```python
from build123d import *

# Parameters (mm, degrees)
SKETCH1_R           = 11
SKETCH1_R_2         = 1.5
SKETCH1_R_3         = 4
BOSS_EXTRUDE1_DEPTH = 16
SKETCH1_4_R         = 11
SKETCH1_4_R_2       = 8
BOSS_EXTRUDE2_DEPTH = 9
SKETCH2_R           = 4
CUT_EXTRUDE1_DEPTH  = 204.169017313
SKETCH3_R           = 4
CUT_EXTRUDE2_DEPTH  = 204.169017313
SKETCH1_5_R         = 11
SKETCH1_5_R_2       = 8
BOSS_EXTRUDE3_DEPTH = 9
CUT_EXTRUDE3_DEPTH  = 2.5
SKETCH5_R           = 4
BOSS_EXTRUDE4_DEPTH = 40
SKETCH6_R           = 4
BOSS_EXTRUDE5_DEPTH = 40


with BuildPart() as part:
    # Sketch1 → Boss-Extrude1 (new body)
    with BuildSketch(Plane(origin=(0, 0, 0), x_dir=(1, 0, 0), z_dir=(0, 1, 0))):
        with BuildLine():
            Line((196.404615305, 34.409093194), (187.656854249, 43.156854249))
            ThreePointArc((187.656854249, 43.156854249), (178.938532541, 44.89103626), (174, 37.5))
            Line((174, 37.5), (174, 24))
            ThreePointArc((174, 24), (171.656854249, 18.343145751), (166, 16))
            Line((166, 16), (150, 16))
            ThreePointArc((150, 16), (145.757359313, 14.242640687), (144, 10))
            Line((144, 10), (144, -10))
            ThreePointArc((144, -10), (145.757359313, -14.242640687), (150, -16))
            Line((150, -16), (166, -16))
            ThreePointArc((166, -16), (171.656854249, -18.343145751), (174, -24))
            Line((174, -24), (174, -37.5))
            ThreePointArc((174, -37.5), (178.938532541, -44.89103626), (187.656854249, -43.156854249))
            Line((187.656854249, -43.156854249), (196.404615305, -34.409093194))
            Line((196.404615305, -34.409093194), (209.37167645, -47.376154339))
            Line((209.37167645, -47.376154339), (237.655947698, -19.091883092))
            Line((237.655947698, -19.091883092), (220, -1.435935394))
            Line((220, -1.435935394), (220, 1.435935394))
            Line((220, 1.435935394), (237.655947698, 19.091883092))
            Line((237.655947698, 19.091883092), (209.37167645, 47.376154339))
            Line((209.37167645, 47.376154339), (196.404615305, 34.409093194))
        make_face()
        with Locations(Location((160, 0, 0), (0, 0, 270))):
            Circle(SKETCH1_R, mode=Mode.SUBTRACT)
        with Locations(Location((150, 10, 0), (0, 0, 270))):
            Circle(SKETCH1_R_2, mode=Mode.SUBTRACT)
        with Locations(Location((170, 10, 0), (0, 0, 270))):
            Circle(SKETCH1_R_2, mode=Mode.SUBTRACT)
        with Locations(Location((170, -10, 0), (0, 0, 270))):
            Circle(SKETCH1_R_2, mode=Mode.SUBTRACT)
        with Locations(Location((150, -10, 0), (0, 0, 270))):
            Circle(SKETCH1_R_2, mode=Mode.SUBTRACT)
        with Locations(Location((204, 0, 0), (0, 0, 270))):
            Circle(SKETCH1_R, mode=Mode.SUBTRACT)
        with Locations(Location((182, 37.5, 0), (0, 0, 270))):
            Circle(SKETCH1_R_3, mode=Mode.SUBTRACT)
        with Locations(Location((194, 10, 0), (0, 0, 270))):
            Circle(SKETCH1_R_2, mode=Mode.SUBTRACT)
        with Locations(Location((214, 10, 0), (0, 0, 270))):
            Circle(SKETCH1_R_2, mode=Mode.SUBTRACT)
        with Locations(Location((214, -10, 0), (0, 0, 270))):
            Circle(SKETCH1_R_2, mode=Mode.SUBTRACT)
        with Locations(Location((194, -10, 0), (0, 0, 270))):
            Circle(SKETCH1_R_2, mode=Mode.SUBTRACT)
        with Locations(Location((182, -37.5, 0), (0, 0, 270))):
            Circle(SKETCH1_R_3, mode=Mode.SUBTRACT)
    extrude(amount=BOSS_EXTRUDE1_DEPTH)

    # Sketch1<4> → Boss-Extrude2 (add)
    with BuildSketch(Plane(origin=(0, 0, 0), x_dir=(1, 0, 0), z_dir=(0, 1, 0))):
        with Locations(Location((204, 0, 0), (0, 0, 270))):
            Circle(SKETCH1_4_R)
        with Locations(Location((204, 0, 0), (0, 0, 270))):
            Circle(SKETCH1_4_R_2, mode=Mode.SUBTRACT)
    extrude(amount=BOSS_EXTRUDE2_DEPTH)

    # Sketch2 → Cut-Extrude1 (cut, through all)
    with BuildSketch(Plane(origin=(109.282032303, 0, 109.282032303), x_dir=(0.7071067811865286, 0, -0.7071067811865666), z_dir=(0.7071067811865666, 0, 0.7071067811865286))):
        with Locations((173.548132206, 8)):
            Circle(SKETCH2_R)
    extrude(amount=-CUT_EXTRUDE1_DEPTH, mode=Mode.SUBTRACT)

    # Sketch3 → Cut-Extrude2 (cut, through all)
    with BuildSketch(Plane(origin=(109.282032303, 0, -109.282032303), x_dir=(-0.7071067811865511, 0, -0.707106781186544), z_dir=(0.707106781186544, 0, -0.7071067811865511))):
        with Locations((-173.548132206, 8)):
            Circle(SKETCH3_R)
    extrude(amount=-CUT_EXTRUDE2_DEPTH, mode=Mode.SUBTRACT)

    # Sketch1<5> → Boss-Extrude3 (add)
    with BuildSketch(Plane(origin=(0, 0, 0), x_dir=(1, 0, 0), z_dir=(0, 1, 0))):
        with Locations(Location((160, 0, 0), (0, 0, 270))):
            Circle(SKETCH1_5_R)
        with Locations(Location((160, 0, 0), (0, 0, 270))):
            Circle(SKETCH1_5_R_2, mode=Mode.SUBTRACT)
    extrude(amount=BOSS_EXTRUDE3_DEPTH)

    # Sketch4 → Cut-Extrude3 (cut)
    with BuildSketch(Plane.XZ):
        Polygon((153.464101615, 10), (151.732050808, 13), (148.267949192, 13), (146.535898385, 10), (148.267949192, 7), (151.732050808, 7), align=None)
        Polygon((173.464101615, 10), (171.732050808, 13), (168.267949192, 13), (166.535898385, 10), (168.267949192, 7), (171.732050808, 7), align=None)
        Polygon((153.464101615, -10), (151.732050808, -7), (148.267949192, -7), (146.535898385, -10), (148.267949192, -13), (151.732050808, -13), align=None)
        Polygon((173.464101615, -10), (171.732050808, -7), (168.267949192, -7), (166.535898385, -10), (168.267949192, -13), (171.732050808, -13), align=None)
        Polygon((197.464101615, 10), (195.732050808, 13), (192.267949192, 13), (190.535898385, 10), (192.267949192, 7), (195.732050808, 7), align=None)
        Polygon((217.464101615, 10), (215.732050808, 13), (212.267949192, 13), (210.535898385, 10), (212.267949192, 7), (215.732050808, 7), align=None)
        Polygon((197.464101615, -10), (195.732050808, -7), (192.267949192, -7), (190.535898385, -10), (192.267949192, -13), (195.732050808, -13), align=None)
        Polygon((217.464101615, -10), (215.732050808, -7), (212.267949192, -7), (210.535898385, -10), (212.267949192, -13), (215.732050808, -13), align=None)
    extrude(amount=-CUT_EXTRUDE3_DEPTH, mode=Mode.SUBTRACT)

    # Sketch5 → Boss-Extrude4 (add)
    with BuildSketch(Plane(origin=(80.997761055, 0, -80.997761055), x_dir=(0.7071067811865509, 0, 0.7071067811865441), z_dir=(-0.7071067811865441, 0, 0.7071067811865509))):
        with BuildLine():
            Line((181.548132206, 16), (181.548132206, 23))
            ThreePointArc((181.548132206, 23), (173.548132206, 31), (165.548132206, 23))
            Line((165.548132206, 23), (165.548132206, 16))
            Line((165.548132206, 16), (181.548132206, 16))
        make_face()
        with Locations((173.548132206, 23)):
            Circle(SKETCH5_R, mode=Mode.SUBTRACT)
    extrude(amount=-BOSS_EXTRUDE4_DEPTH)

    # Sketch6 → Boss-Extrude5 (add)
    with BuildSketch(Plane(origin=(80.997761055, 0, 80.997761055), x_dir=(-0.7071067811865172, 0, 0.707106781186578), z_dir=(-0.707106781186578, 0, -0.7071067811865172))):
        with BuildLine():
            Line((-165.548132206, 16), (-165.548132206, 23))
            ThreePointArc((-165.548132206, 23), (-173.548132206, 31), (-181.548132206, 23))
            Line((-181.548132206, 23), (-181.548132206, 16))
            Line((-181.548132206, 16), (-165.548132206, 16))
        make_face()
        with Locations((-173.548132206, 23)):
            Circle(SKETCH6_R, mode=Mode.SUBTRACT)
    extrude(amount=-BOSS_EXTRUDE5_DEPTH)


solid = part.part
```
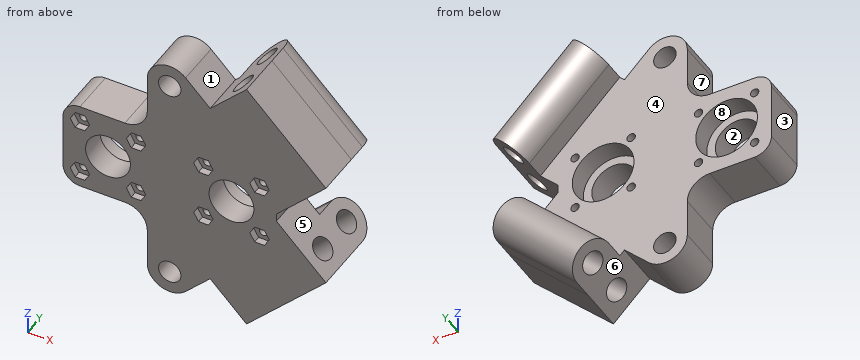
Geometry check sheet. Reference: the model listing, model coordinates, mm. Face numbers are marked on the shaded views. A direction names the side the tool comes from. Coordinates: 2 decimals unless noted, no trailing zeros. Loops run counter-clockwise (first coordinate to the right, second up) from the corner with the lowest first, then second, coordinate; pieces in that order, holes last. Notation, with made-up numbers: (10, 50) - (27, 50) arc R21 cw to (27, 57) - close; hole circle Ø3 at (-5, 45.25). An arc over 180 degrees is marked (long way). One line per item, written item: value. Start each with the question number.
(1) Material ranges on line 1 (X direction, y = 4, z = 0); line 2 (X direction, y = 6.5, z = -10.5); line 3 (Z direction, x = 194, y = 5), recorded low to high. Write a range as [from, to].
(2) Depth check by flat-ended pin: P1, Ø13, axis at x = 160, z = 0, coming from the +Y side; P2, Ø2, axis at x = 214.5, y = 1, coming from the -Z side; P3, Ø10, axis at x = 154, z = -7.5, coming from the +Y side; P4, Ø3.5, axis at x = 194, z = -10, coming from the -Y side. Enter the tip coordinate at first touch or a pass-through.
(3) Cross-section at D-D on y = 29. Enter the section's corners in (x, z).
(4) Cross-section at C-C on y = 14.5. Count the separate pieces of the cut face and the enclosed holes in it, plus the area to 3 significant figures.
(5) Mould release check, pull along Z, two halves, no side actions. Record for the marked faces 1, 2 and 3: released by +Z, released by -Z, zero draft, split by the parting line, or undercut.
(6) Tool access check on the marked faces 4, 5, 6, 7 and 8. Record the directions out of +Z, -Z, +X, -X, +Y, -Y that give a thin tool (end or side, any length) a straight path to the whole face; none if there is none.
(7) Cross-section at B-B on z = 0. Enter the section's corners in (x, y).
(8) Cross-section at A-A on x = 160. Enter the section's corners in (y, z), plus the area to 3 significant figures.
Results below:
1. line 1: x = [144, 152], [168, 196], [212, 220]
1. line 2: x = [144.02, 148.59], [151.41, 168.59], [171.41, 192.59], [195.41, 212.59], [215.41, 229.06]
1. line 3: z = [-36.81, -11.5], [-8.5, 8.5], [11.5, 36.81]
2. P1: passes through
2. P2: stops at z = -43.25
2. P3: stops at y = 16
2. P4: stops at y = 2.5
3. outline: (199.97, -37.98) - (207.46, -45.46) - (235.74, -17.18) - (228.26, -9.69) - close; (199.97, 37.98) - (228.26, 9.69) - (235.74, 17.18) - (207.46, 45.46) - close
4. separate pieces: 1
4. enclosed holes: 12
4. area: 4,520 mm2
5. face 1: released by +Z
5. face 2: undercut
5. face 3: zero draft
6. face 4: -X, +Y
6. face 5: +X, +Y, -Y
6. face 6: -Z, +Y, -Y
6. face 7: +Z, -X, +Y, -Y
6. face 8: +Y
7. outline: (144, 0) - (152, 0) - (152, 9) - (149, 9) - (149, 16) - (144, 16) - close; (168, 0) - (196, 0) - (196, 9) - (193, 9) - (193, 16) - (171, 16) - (171, 9) - (168, 9) - close; (212, 0) - (220, 0) - (220, 16) - (215, 16) - (215, 9) - (212, 9) - close
8. outline: (0, -16) - (16, -16) - (16, -11) - (9, -11) - (9, -8) - (0, -8) - close; (0, 8) - (9, 8) - (9, 11) - (16, 11) - (16, 16) - (0, 16) - close
8. area: 214 mm2
